Source: CAD feature listing. Evaluate the final solid. Frame: model axes, mm. A direction names the side the tool comes from. Coordinates: 2 decimals unless noted, no trailing zeros. Order: outer loops, then holes, each group sorted by start corner. A loop starts at its lowest first (then second) coordinate and runs counter-clockwise, first axis right, second up. Notation, with made-up numbers: (-22.5, 79) - (29.5, 79) arc R14 ccw to (29.5, 95) - close; hole circle Ø4 at (-33, -8.75). An arc over 180 degrees is marked (long way). One line per question, with ' | ' between items.
from build123d import *

# Parameters (mm, degrees)
RESSALTO_EXTRUS_O2_DEPTH = 9.2
ESBO_O5_R                = 2.15
CORTE_EXTRUS_O2_DEPTH    = 9.2
CHANFRO2_SIZE            = 0.3
SKETCH1_W                = 40
SKETCH1_H                = 3.972261678
BOSS_EXTRUDE1_DEPTH      = 10
SKETCH2_W                = 40
SKETCH2_H                = 6
BOSS_EXTRUDE2_DEPTH      = 38.1


with BuildPart() as part:
    # Esboço4 → Ressalto-extrusão2 (new body)
    with BuildSketch(Plane(origin=(0, 0, 0), x_dir=(1, 0, 0), z_dir=(0, 1, 0))):
        with BuildLine():
            Line((-19.2, 2.35), (-19.2, 1.65))
            ThreePointArc((-19.2, 1.65), (-19.170710678, 1.579289322), (-19.1, 1.55))
            Line((-19.1, 1.55), (-18.1, 1.55))
            ThreePointArc((-18.1, 1.55), (-18.029289322, 1.579289322), (-18, 1.65))
            Line((-18, 1.65), (-18, 2.35))
            ThreePointArc((-18, 2.35), (-17.970710678, 2.420710678), (-17.9, 2.45))
            Line((-17.9, 2.45), (-17.3, 2.45))
            ThreePointArc((-17.3, 2.45), (-17.229289322, 2.420710678), (-17.2, 2.35))
            Line((-17.2, 2.35), (-17.2, 1.65))
            ThreePointArc((-17.2, 1.65), (-17.170710678, 1.579289322), (-17.1, 1.55))
            Line((-17.1, 1.55), (-16.1, 1.55))
            ThreePointArc((-16.1, 1.55), (-16.029289322, 1.579289322), (-16, 1.65))
            Line((-16, 1.65), (-16, 2.35))
            ThreePointArc((-16, 2.35), (-15.970710678, 2.420710678), (-15.9, 2.45))
            Line((-15.9, 2.45), (-15.3, 2.45))
            ThreePointArc((-15.3, 2.45), (-15.229289322, 2.420710678), (-15.2, 2.35))
            Line((-15.2, 2.35), (-15.2, 1.65))
            ThreePointArc((-15.2, 1.65), (-15.170710678, 1.579289322), (-15.1, 1.55))
            Line((-15.1, 1.55), (-14.1, 1.55))
            ThreePointArc((-14.1, 1.55), (-14.029289322, 1.579289322), (-14, 1.65))
            Line((-14, 1.65), (-14, 2.35))
            ThreePointArc((-14, 2.35), (-13.970710678, 2.420710678), (-13.9, 2.45))
            Line((-13.9, 2.45), (-13.3, 2.45))
            ThreePointArc((-13.3, 2.45), (-13.229289322, 2.420710678), (-13.2, 2.35))
            Line((-13.2, 2.35), (-13.2, 1.65))
            ThreePointArc((-13.2, 1.65), (-13.170710678, 1.579289322), (-13.1, 1.55))
            Line((-13.1, 1.55), (-12.1, 1.55))
            ThreePointArc((-12.1, 1.55), (-12.029289322, 1.579289322), (-12, 1.65))
            Line((-12, 1.65), (-12, 2.35))
            ThreePointArc((-12, 2.35), (-11.970710678, 2.420710678), (-11.9, 2.45))
            Line((-11.9, 2.45), (-11.3, 2.45))
            ThreePointArc((-11.3, 2.45), (-11.229289322, 2.420710678), (-11.2, 2.35))
            Line((-11.2, 2.35), (-11.2, 1.65))
            ThreePointArc((-11.2, 1.65), (-11.170710678, 1.579289322), (-11.1, 1.55))
            Line((-11.1, 1.55), (-10.1, 1.55))
            ThreePointArc((-10.1, 1.55), (-10.029289322, 1.579289322), (-10, 1.65))
            Line((-10, 1.65), (-10, 2.35))
            ThreePointArc((-10, 2.35), (-9.970710678, 2.420710678), (-9.9, 2.45))
            Line((-9.9, 2.45), (-9.3, 2.45))
            ThreePointArc((-9.3, 2.45), (-9.229289322, 2.420710678), (-9.2, 2.35))
            Line((-9.2, 2.35), (-9.2, 1.65))
            ThreePointArc((-9.2, 1.65), (-9.170710678, 1.579289322), (-9.1, 1.55))
            Line((-9.1, 1.55), (-8.1, 1.55))
            ThreePointArc((-8.1, 1.55), (-8.029289322, 1.579289322), (-8, 1.65))
            Line((-8, 1.65), (-8, 2.35))
            ThreePointArc((-8, 2.35), (-7.970710678, 2.420710678), (-7.9, 2.45))
            Line((-7.9, 2.45), (-7.3, 2.45))
            ThreePointArc((-7.3, 2.45), (-7.229289322, 2.420710678), (-7.2, 2.35))
            Line((-7.2, 2.35), (-7.2, 1.65))
            ThreePointArc((-7.2, 1.65), (-7.170710678, 1.579289322), (-7.1, 1.55))
            Line((-7.1, 1.55), (7.1, 1.55))
            ThreePointArc((7.1, 1.55), (7.170710678, 1.579289322), (7.2, 1.65))
            Line((7.2, 1.65), (7.2, 2.35))
            ThreePointArc((7.2, 2.35), (7.229289322, 2.420710678), (7.3, 2.45))
            Line((7.3, 2.45), (7.9, 2.45))
            ThreePointArc((7.9, 2.45), (7.970710678, 2.420710678), (8, 2.35))
            Line((8, 2.35), (8, 1.65))
            ThreePointArc((8, 1.65), (8.029289322, 1.579289322), (8.1, 1.55))
            Line((8.1, 1.55), (9.1, 1.55))
            ThreePointArc((9.1, 1.55), (9.170710678, 1.579289322), (9.2, 1.65))
            Line((9.2, 1.65), (9.2, 2.35))
            ThreePointArc((9.2, 2.35), (9.229289322, 2.420710678), (9.3, 2.45))
            Line((9.3, 2.45), (9.9, 2.45))
            ThreePointArc((9.9, 2.45), (9.970710678, 2.420710678), (10, 2.35))
            Line((10, 2.35), (10, 1.65))
            ThreePointArc((10, 1.65), (10.029289322, 1.579289322), (10.1, 1.55))
            Line((10.1, 1.55), (11.1, 1.55))
            ThreePointArc((11.1, 1.55), (11.170710678, 1.579289322), (11.2, 1.65))
            Line((11.2, 1.65), (11.2, 2.35))
            ThreePointArc((11.2, 2.35), (11.229289322, 2.420710678), (11.3, 2.45))
            Line((11.3, 2.45), (11.9, 2.45))
            ThreePointArc((11.9, 2.45), (11.970710678, 2.420710678), (12, 2.35))
            Line((12, 2.35), (12, 1.65))
            ThreePointArc((12, 1.65), (12.029289322, 1.579289322), (12.1, 1.55))
            Line((12.1, 1.55), (13.1, 1.55))
            ThreePointArc((13.1, 1.55), (13.170710678, 1.579289322), (13.2, 1.65))
            Line((13.2, 1.65), (13.2, 2.35))
            ThreePointArc((13.2, 2.35), (13.229289322, 2.420710678), (13.3, 2.45))
            Line((13.3, 2.45), (13.9, 2.45))
            ThreePointArc((13.9, 2.45), (13.970710678, 2.420710678), (14, 2.35))
            Line((14, 2.35), (14, 1.65))
            ThreePointArc((14, 1.65), (14.029289322, 1.579289322), (14.1, 1.55))
            Line((14.1, 1.55), (15.1, 1.55))
            ThreePointArc((15.1, 1.55), (15.170710678, 1.579289322), (15.2, 1.65))
            Line((15.2, 1.65), (15.2, 2.35))
            ThreePointArc((15.2, 2.35), (15.229289322, 2.420710678), (15.3, 2.45))
            Line((15.3, 2.45), (15.9, 2.45))
            ThreePointArc((15.9, 2.45), (15.970710678, 2.420710678), (16, 2.35))
            Line((16, 2.35), (16, 1.65))
            ThreePointArc((16, 1.65), (16.029289322, 1.579289322), (16.1, 1.55))
            Line((16.1, 1.55), (17.1, 1.55))
            ThreePointArc((17.1, 1.55), (17.170710678, 1.579289322), (17.2, 1.65))
            Line((17.2, 1.65), (17.2, 2.35))
            ThreePointArc((17.2, 2.35), (17.229289322, 2.420710678), (17.3, 2.45))
            Line((17.3, 2.45), (17.9, 2.45))
            ThreePointArc((17.9, 2.45), (17.970710678, 2.420710678), (18, 2.35))
            Line((18, 2.35), (18, 1.65))
            ThreePointArc((18, 1.65), (18.029289322, 1.579289322), (18.1, 1.55))
            Line((18.1, 1.55), (19.1, 1.55))
            ThreePointArc((19.1, 1.55), (19.170710678, 1.579289322), (19.2, 1.65))
            Line((19.2, 1.65), (19.2, 2.35))
            ThreePointArc((19.2, 2.35), (19.229289322, 2.420710678), (19.3, 2.45))
            Line((19.3, 2.45), (19.9, 2.45))
            ThreePointArc((19.9, 2.45), (19.970710678, 2.420710678), (20, 2.35))
            Line((20, 2.35), (20, -2.45))
            Line((20, -2.45), (-20, -2.45))
            Line((-20, -2.45), (-20, 2.35))
            ThreePointArc((-20, 2.35), (-19.970710678, 2.420710678), (-19.9, 2.45))
            Line((-19.9, 2.45), (-19.3, 2.45))
            ThreePointArc((-19.3, 2.45), (-19.229289322, 2.420710678), (-19.2, 2.35))
        make_face()
    extrude(amount=RESSALTO_EXTRUS_O2_DEPTH)

    # Esboço5 → Corte-extrusão2 (cut)
    with BuildSketch(Plane(origin=(0, 0, -1.55), x_dir=(-1, 0, 0), z_dir=(0, 0, -1))):
        with Locations((0, 4.6)):
            Circle(ESBO_O5_R)
    extrude(amount=-CORTE_EXTRUS_O2_DEPTH, mode=Mode.SUBTRACT)

    # Chanfro2
    chanfro2_edges = [part.edges().sort_by_distance(p)[0] for p in [
        (2.15, 4.6, -1.55),
    ]]
    chamfer(chanfro2_edges, length=CHANFRO2_SIZE)

    # Sketch1 → Boss-Extrude1 (add)
    with BuildSketch(Plane(origin=(0, 9.2, 0), x_dir=(1, 0, 0), z_dir=(0, 1, 0))):
        with Locations((0, -0.463869161)):
            Rectangle(SKETCH1_W, SKETCH1_H)
    extrude(amount=BOSS_EXTRUDE1_DEPTH)

    # Sketch2 → Boss-Extrude2 (add)
    with BuildSketch(Plane.XY.offset(2.45)):
        with Locations((0, 16.2)):
            Rectangle(SKETCH2_W, SKETCH2_H)
    extrude(amount=BOSS_EXTRUDE2_DEPTH)


solid = part.part
(1) Cut plane D-D (z = 11). Return the cut outline in (x, y).
Taken from the geometry:
outline: (-20, 13.2) - (20, 13.2) - (20, 19.2) - (-20, 19.2) - close
(2) Cut plane A-A (z = 1.5). Return the cut outline in (x, y), and give its area (3 significant figures).
Taken from the geometry:
outline: (-20, 0) - (20, 0) - (20, 19.2) - (-20, 19.2) - close; hole circle Ø4.3 at (0, 4.6) | area: 753 mm²
(3) Set-up query: faces 1 (the flat face through (0, 8, 2.45)), 2 (the flat face through (7.5, 9.2, -2)), 3 (the flat face through (10.6, 4.5, -1.55)). Return all of +Z, -Z, +X, -X, +Y, -Y with unobstructed straight access to the full face (end or side cutting, diameter ignored); none if empty.
Taken from the geometry:
face 1: +Z, +X, -X, -Y | face 2: -Z, +X, -X, +Y | face 3: -Z, +Y, -Y
(4) Cut plane C-C (y = 15.5). Return the cut outline in (x, z), and give its area (3 significant figures).
Taken from the geometry:
outline: (-20, -1.52) - (20, -1.52) - (20, 40.55) - (-20, 40.55) - close | area: 1,680 mm²
(5) Pull-direction query (Y, two-part tool) for faces 4 (the flat face through (0, 13.2, 21)), 5 (the flat face through (18.6, 4.5, -1.55)), 6 (the cylindrical face through (0.47, 2.5, 0.57)); classes: pulls with the +Y half, pulls with the -Y half, needs draft (parallel to the pull), parting line crosses it, or undercut.
Taken from the geometry:
face 4: pulls with the -Y half | face 5: needs draft | face 6: undercut
(6) Pin query (flat end, axial travel): P1, Ø1, axis at x = 5.5, z = 31, coming from the -Y side; P2, Ø1, axis at x = 0.5, y = 11, coming from the -Z side; P3, Ø0.8, axis at x = -12.5, y = 6.5, coming from the -Z side. Return the tip coordinate at first contact, or that it passes through.
Taken from the geometry:
P1: stops at y = 13.2 | P2: stops at z = -1.52 | P3: stops at z = -1.55
(7) Material intervals for L1, parallel to Y at x = 0, z = -0.3; L2, parallel to Y at x = -5, z = 27; L3, parallel to Z at x = 9, y = 8.5, sorted ascending. Write a range as from..to.
Taken from the geometry:
L1: y = 0..2.45, 6.75..19.2 | L2: y = 13.2..19.2 | L3: z = -1.55..2.45
